Autodesk Inventor part; units mm, degrees
ref_plane "YZ Plane" through (0, 0, 0) normal (1, 0, 0) x (0, 1, 0)
ref_plane "XZ Plane" through (0, 0, 0) normal (0, 1, 0) x (-1, 0, 0)
ref_plane "XY Plane" through (0, 0, 0) normal (0, 0, 1) x (1, 0, 0)
sketch "Sketch1" plane through (0, 0, 0) normal (0, 1, 0) x (-1, 0, 0)
  circle A0 centre (0, 0) radius 2
  circle A1 centre (0, 0) radius 4.5
  dimension "d0" = 4
  dimension "d1" = 9
extrude "Extrusion1" add sketch "Sketch1" along normal blind 4
sketch "Sketch2" plane through (0, 4, 0) normal (0, 1, 0) x (1, 0, 0)
  circle A0 centre (0, 0) radius 4.5
  circle A1 centre (0, 0) radius 2
  circle A2 centre (0, 0) radius 2.5
  circle A3 centre (0, 0) radius 2
  circle A4 centre (0, 0) radius 4
  dimension "d4" = 5
  dimension "d5" = 8
extrude "Extrusion2" cut sketch "Sketch2" against normal blind 0.1 contours A4
sketch "Sketch3" plane through (0, 0, 0) normal (0, -1, 0) x (1, 0, 0)
  circle A0 centre (0, 0) radius 4
  circle A1 centre (0, 0) radius 2.5
extrude "Extrusion3" cut sketch "Sketch3" against normal blind 0.1
properties part number "bearing_4_9_4"
Check sheet for the modelled part. Datum: model origin and axes. Units: mm. A direction names the side the tool comes from. Round coordinates to 2 decimals unless told otherwise and drop trailing zeros. Write each loop counter-clockwise with the first axis right and the second up, starting at its lowest first coordinate (ties: lowest second). Pieces come first, ordered by that corner, then holes. Notation, with made-up numbers: (43, 79) - (94, 79) arc R14 ccw to (94, 100) - close; hole circle Ø8 at (-7.75, 41). An arc over 180 degrees is marked (long way). Return JSON: item names as keys, results as strings.
Q1. Cross-section at B-B (x = 0). Record the boundary of the cut face in (y, z), then the cut area to 3 significant figures.
Returned:
{"outline": "(0, -4.5) - (4, -4.5) - (4, -4) - (3.9, -4) - (3.9, -2.5) - (4, -2.5) - (4, -2) - (0, -2) - (0, -2.5) - (0.1, -2.5) - (0.1, -4) - (0, -4) - close; (0, 2) - (4, 2) - (4, 2.5) - (3.9, 2.5) - (3.9, 4) - (4, 4) - (4, 4.5) - (0, 4.5) - (0, 4) - (0.1, 4) - (0.1, 2.5) - (0, 2.5) - close", "area": "19.4 mm²"}
Q2. Depth check by flat-ended pin: P1, Ø5, axis at x = -3, z = -2, coming from the +Y side; P2, Ø2, axis at y = 3.5, z = -3.5, coming from the -X side. Enter the tip coordinate at first touch or a pass-through.
Returned:
{"P1": "stops at y = 4", "P2": "stops at x = -3.74"}
Q3. Cross-section at A-A (z = 0). Record the boundary of the cut face in (x, y).
Returned:
{"outline": "(-4.5, 0) - (-4, 0) - (-4, 0.1) - (-2.5, 0.1) - (-2.5, 0) - (-2, 0) - (-2, 4) - (-2.5, 4) - (-2.5, 3.9) - (-4, 3.9) - (-4, 4) - (-4.5, 4) - close; (2, 0) - (2.5, 0) - (2.5, 0.1) - (4, 0.1) - (4, 0) - (4.5, 0) - (4.5, 4) - (4, 4) - (4, 3.9) - (2.5, 3.9) - (2.5, 4) - (2, 4) - close"}
Q4. Cross-section at D-D (z = -3.5). Record the boundary of the cut face in (x, y), then the cut area to 3 significant figures.
Returned:
{"outline": "(-2.83, 0) - (-1.94, 0) - (-1.94, 0.1) - (1.94, 0.1) - (1.94, 0) - (2.83, 0) - (2.83, 4) - (1.94, 4) - (1.94, 3.9) - (-1.94, 3.9) - (-1.94, 4) - (-2.83, 4) - close", "area": "21.9 mm²"}
Q5. Access from +Z, -Z, +X, -X, +Y, -Y to the whole of each face (thin tool, end or side, straight path). Record for faces 1 (the flat face through (1, 0, 2)), 2 (the flat face through (2, 3.9, -2)).
Returned:
{"face 1": "+Z, -Z, +X, -X, -Y", "face 2": "+Y"}
Q6. Draft check along X on faces 3 (the flat face through (3, 4, -3)), 4 (the cylindrical face through (0.59, 1.97, -4.46)), 5 (the flat face through (2, 0.1, 2)). Enter one of: released by +X, released by -X, zero draft, split by the parting line, or undercut.
Returned:
{"face 3": "zero draft", "face 4": "split by the parting line", "face 5": "undercut"}
Q7. Cross-section at C-C (y = 1.25). Record the boundary of the cut face in (x, z), then the cut area to 3 significant figures.
Returned:
{"outline": "circle Ø9 at (0, 0); hole circle Ø4 at (0, 0)", "area": "51.1 mm²"}
Q8. Scan lines: L1, parallel to Z at x = 0, y = 0.15; L2, parallel to Z at x = 1.5, y = 2.2; L3, parallel to X at y = 1.8, z = 1.75. Record each from-to range of solid material in increasing order. Write a range as from..to.
Returned:
{"L1": "z = -4.5..-2, 2..4.5", "L2": "z = -4.24..-1.32, 1.32..4.24", "L3": "x = -4.15..-0.97, 0.97..4.15"}
